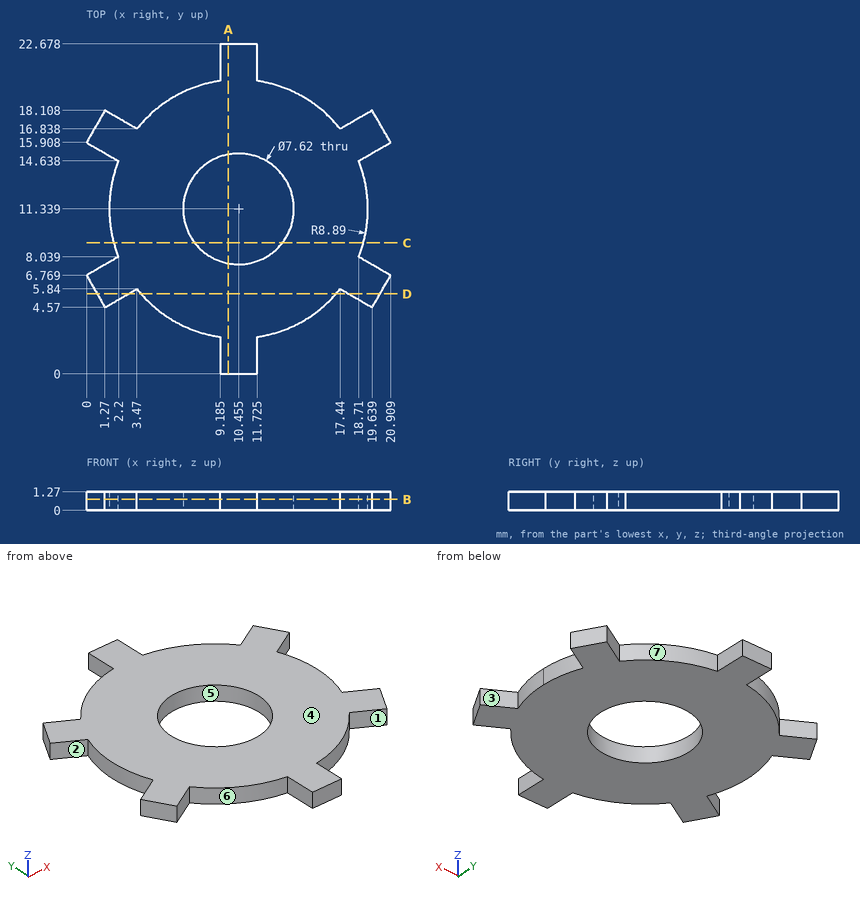
Design review of the part shown in the three views and the two pictorial views. Dimensions are in mm from the part's minimum x, y and z. A direction names the side the tool comes from. Round coordinates to 2 decimals unless told otherwise and drop trailing zeros. Loops run counter-clockwise (first coordinate to the right, second up) from the corner with the lowest first, then second, coordinate; pieces in that order, holes last. Notation, with made-up numbers: (-8.75, -1) - (16.25, -1) arc R28 cw to (16.25, 27) - close; hole circle Ø1 at (65.5, 38.5). An arc over 180 degrees is marked (long way). Use one line per item in the form item = value.
1) We need section A-A on x = 9.75. Write out the cut boundary in (y, z) (1 decimal).
Solutions:
outline = (0, 0) - (7.6, 0) - (7.6, 1.3) - (0, 1.3) - close; (15.1, 0) - (22.7, 0) - (22.7, 1.3) - (15.1, 1.3) - close
2) Clearance check with a flat-ended pin moving along its axis: P1, Ø0.6, axis at y = 1.5, z = 0.5, coming from the -X side (1 decimal). State where the tip first meets the part, or that it passes through.
Solutions:
P1 = 9.2
3) Tool access review of the marked faces 5, 6 and 7: name each direction out of +Z, -Z, +X, -X, +Y, -Y from which nothing blocks a thin tool from reaching the whole face with its end or side.
Solutions:
face_5 = +Z, -Z
face_6 = +Z, -Z, -Y
face_7 = +Z, -Z, +Y
4) We need section B-B on z = 0.75. Write out the cut boundary in (x, y) (1 decimal).
Solutions:
outline = (0, 6.8) - (1.3, 4.6) - (3.5, 5.8) arc R8.9 ccw to (9.2, 2.5) - (9.2, 0) - (11.7, 0) - (11.7, 2.5) arc R8.9 ccw to (17.4, 5.8) - (19.6, 4.6) - (20.9, 6.8) - (18.7, 8) arc R8.9 ccw to (19.3, 11.3) arc R8.9 ccw to (18.7, 14.6) - (20.9, 15.9) - (19.6, 18.1) - (17.4, 16.8) arc R8.9 ccw to (11.7, 20.1) - (11.7, 22.7) - (9.2, 22.7) - (9.2, 20.1) arc R8.9 ccw to (3.5, 16.8) - (1.3, 18.1) - (0, 15.9) - (2.2, 14.6) arc R8.9 ccw to (2.2, 8) - close; hole circle Ø7.6 at (10.5, 11.3)
5) Mouldability with a two-part tool opening along X and no side actions: class the marked faces 1, 2, 3 and 4 as pulls with the +X half, pulls with the -X half, needs draft (parallel to the pull), parting line crosses it, or undercut.
Solutions:
face_1 = undercut
face_2 = pulls with the -X half
face_3 = pulls with the +X half
face_4 = needs draft
6) Wall thickness on probe 1 along X at (y, z) = (11.25, 0.5) (1 decimal); probe 2 along X at (y, z) = (17, 0.9); probe 3 along X at (y, z) = (20.25, 0.15) (1 decimal): over which ranges is each line inside the solid? List them lowest first.
Solutions:
probe_1 = 1.6 to 6.6, 14.3 to 19.3
probe_2 = 0.63 to 3.19, 3.6 to 17.31, 17.72 to 20.28
probe_3 = 9.2 to 11.7
7) We need section D-D on y = 5.5. Write out the cut boundary in (x, z).
Solutions:
outline = (0.73, 0) - (2.88, 0) - (2.88, 1.27) - (0.73, 1.27) - close; (3.75, 0) - (17.16, 0) - (17.16, 1.27) - (3.75, 1.27) - close; (18.03, 0) - (20.18, 0) - (20.18, 1.27) - (18.03, 1.27) - close
8) We need section C-C on y = 9. Write out the cut boundary in (x, z).
Solutions:
outline = (1.88, 0) - (7.45, 0) - (7.45, 1.27) - (1.88, 1.27) - close; (13.46, 0) - (19.03, 0) - (19.03, 1.27) - (13.46, 1.27) - close
